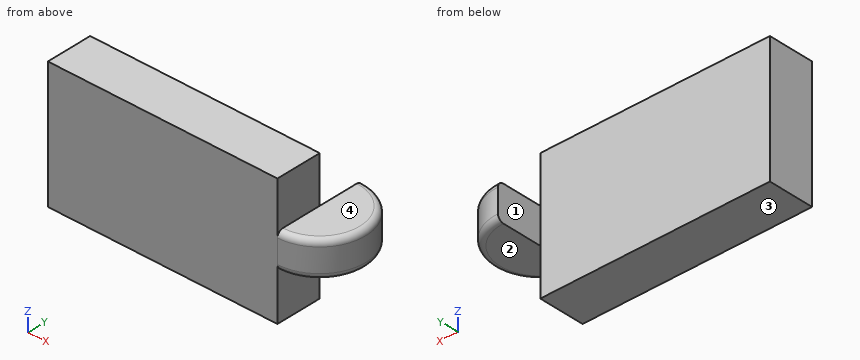
from build123d import *

# Parameters (mm, degrees)
F0_W     = 77.996812
F0_H     = 43.68491
F1_DEPTH = 7.8
F3_DEPTH = 6
F4_R     = 2


with BuildPart() as f1:
    # F0 (on Front) → F1 (new body, symmetric)
    with BuildSketch(Plane.XZ):
        Rectangle(F0_W, F0_H)
    extrude(amount=F1_DEPTH, both=True)

    # F2 (on Top) → F3 (join, symmetric)
    with BuildSketch(Plane.XY):
        with BuildLine():
            Line((38.998406, 7.8), (38.998406, -7.8))
            ThreePointArc((38.998406, -7.8), (54.598406, 7.8), (38.998406, 23.4))
            Line((38.998406, 23.4), (38.998406, 7.8))
        make_face()
    extrude(amount=F3_DEPTH, both=True)

    # F4
    f4_edges = [f1.edges().sort_by_distance(p)[0] for p in [
        (54.598406, 7.8, 6),
        (54.598406, 7.8, -6),
    ]]
    fillet(f4_edges, radius=F4_R)


solid = f1.part
The model under review builds one solid part; all positions refer to its coordinate system, in mm. Face numbers are marked on the shaded views. A direction names the side the tool comes from. Give positions to 0.01 mm unless a question says otherwise; leave off trailing zeros. Loops run counter-clockwise (first coordinate to the right, second up) from the corner with the lowest first, then second, coordinate; pieces in that order, holes last. Notation, with made-up numbers: (-13, 40) -> (36, 40) arc R33 cw to (36, 74) -> close; hole circle Ø3 at (33, 53.5). An arc over 180 degrees is marked (long way). Answer as a JSON object with one key per item and string values. Group by question number.
Q1. Wall thickness on line 1 along Y through (x, z) = (24.5, 3); line 2 along X through (y, z) = (4, -11.5); line 3 along X through (y, z) = (4.5, -2.5): over which ranges is each line inside the solid? List them lowest first.
Q2. Insertion check: pin 1 (4 mm diameter, centred on x = 47, y = 7.5, fed in from -Z); pin 2 (13 mm diameter, centred on y = 15.5, z = 2.5, fed in from -X); pin 3 (22 mm diameter, centred on x = 12, z = -3.5, fed in from +Y). Each pin has a flat end and moves straight along its axis. Give the tip position at first contact, or say it passes through.
Q3. Take a section at A-A (x = 2). Write out the cut boundary in (y, z), plus the area to 3 significant figures.
Q4. Take a section at B-B (z = 9). Write out the cut boundary in (x, y), plus the area to 3 significant figures.
Q5. Tool access review of the marked faces 1, 2, 3 and 4: name each direction out of +Z, -Z, +X, -X, +Y, -Y from which nothing blocks a thin tool from reaching the whole face with its end or side.
Answer below:
{
 "1": {"line 1": "y = -7.8 to 7.8", "line 2": "x = -39 to 39", "line 3": "x = -39 to 54.25"},
 "2": {"pin 1": "stops at z = -6", "pin 2": "stops at x = 39", "pin 3": "stops at y = 7.8"},
 "3": {"outline": "(-7.8, -21.84) -> (7.8, -21.84) -> (7.8, 21.84) -> (-7.8, 21.84) -> close", "area": "681 mm2"},
 "4": {"outline": "(-39, -7.8) -> (39, -7.8) -> (39, 7.8) -> (-39, 7.8) -> close", "area": "1,220 mm2"},
 "5": {"face 1": "+Z, -Z, -X, +Y", "face 2": "-Z, +X, +Y, -Y", "face 3": "-Z, +X, -X, +Y, -Y", "face 4": "+Z, +X, +Y, -Y"}
}
